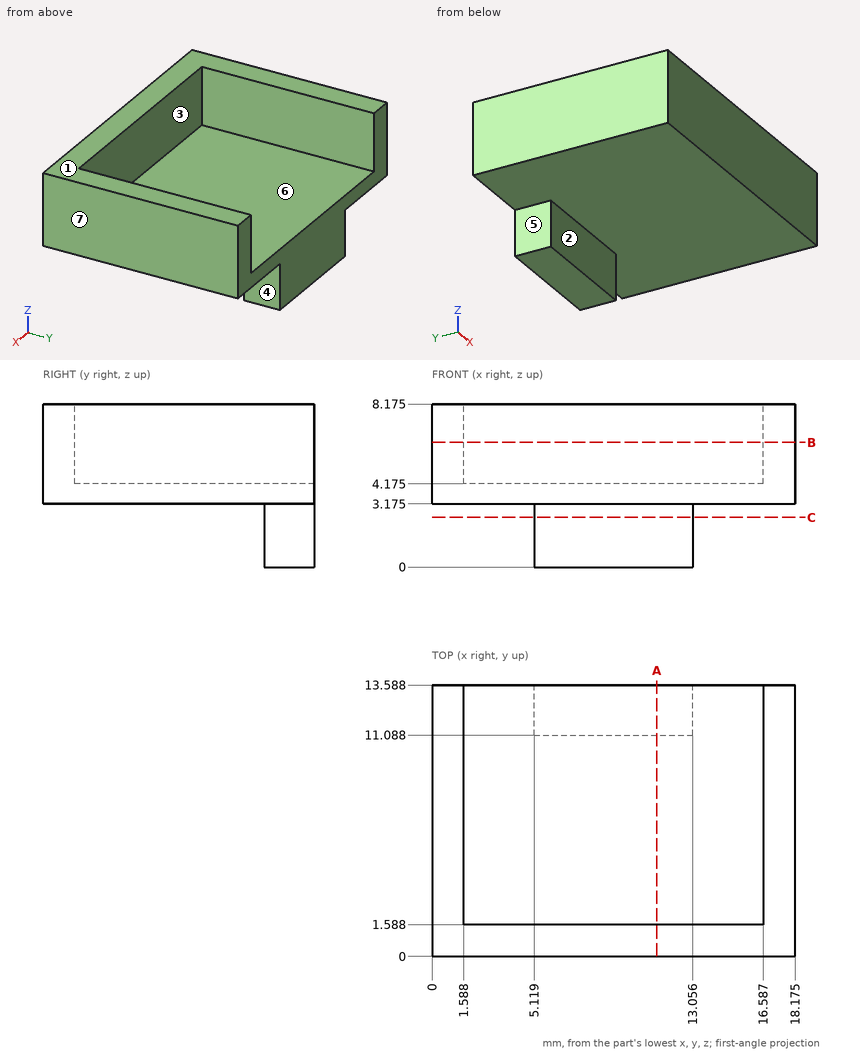
Answer from the drawing. Dimensions are ordinates in mm from the lowest x, y and z of the part. A direction names the side the tool comes from. Give positions to 0.01 mm unless a question says otherwise; leave off trailing zeros. Loops run counter-clockwise (first coordinate to the right, second up) from the corner with the lowest first, then second, coordinate; pieces in that order, holes last.
Item 1: For the marked faces 1, 2, 3 and 4, determine the directions among +Z, -Z, +X, -X, +Y, -Y from which every point of the face is accessible in a straight line to the end or side of a thin tool.
Item 2: Each of these flat-tipped pins is pushed along its axis until it touches: pin 1 Ø2 at (y, z) = (12.5, 2) entering from -X; pin 2 Ø6 at (x, y) = (7.5, 6) entering from -Z (1 decimal); pin 3 Ø3 at (y, z) = (12, 1.5) entering from +X. Where does it stop, or does it pass through?
Item 3: The mould has two halves that part along X. Classify the marked faces 5, 6 and 7: released by +X, released by -X, zero draft, split by the parting line, or undercut.
Item 4: The part is cut by section C-C (z = 2.5). Write down the section's boundary in (x, y).
Item 5: The part is cut by section B-B (z = 6.25). Write down the section's boundary in (x, y) (1 decimal).
Item 6: Find the intervals of material crossed by line 1 along X through (y, z) = (5.75, 4.25) (1 decimal); line 2 along Z through (x, y) = (10, 13) (1 decimal); line 3 along Z through (x, y) = (7.75, 8.5) (1 decimal), in increasing order.
Item 7: The part is cut by section A-A (x = 11.25). Write down the section's boundary in (y, z) (1 decimal).
Taken from the geometry:
1. face 1: +Z, +X, -X, +Y, -Y
1. face 2: -Z, +X, -X, -Y
1. face 3: +Z, +Y
1. face 4: -Z, +X, +Y, -Y
2. pin 1: stops at x = 5.12
2. pin 2: stops at z = 3.2
2. pin 3: stops at x = 13.06
3. face 5: released by -X
3. face 6: undercut
3. face 7: released by +X
4. outline: (5.12, 11.09) - (13.06, 11.09) - (13.06, 13.59) - (5.12, 13.59) - close
5. outline: (0, 0) - (18.2, 0) - (18.2, 13.6) - (16.6, 13.6) - (16.6, 1.6) - (1.6, 1.6) - (1.6, 13.6) - (0, 13.6) - close
6. line 1: x = 0 to 1.6, 16.6 to 18.2
6. line 2: z = 0 to 4.2
6. line 3: z = 3.2 to 4.2
7. outline: (0, 3.2) - (11.1, 3.2) - (11.1, 0) - (13.6, 0) - (13.6, 4.2) - (1.6, 4.2) - (1.6, 8.2) - (0, 8.2) - close
